The model under review builds one solid part; all positions refer to its coordinate system, in mm. Face numbers are marked on the shaded views. Give positions to 0.01 mm unless a question says otherwise; leave off trailing zeros. Write each loop counter-clockwise with the first axis right and the second up, starting at its lowest first coordinate (ties: lowest second). Pieces come first, ordered by that corner, then holes. Notation, with made-up numbers: (-19.5, -5.75) - (18.5, -5.75) arc R30 cw to (18.5, 22.25) - close; hole circle Ø11 at (-8, -2.5). An arc over 180 degrees is marked (long way). Write item = value, one per line.
```python
from build123d import *

# Parameters (mm, degrees)
SKETCH_1_W          = 140
SKETCH_1_H          = 130
EXTRUDE_1_DEPTH     = 60
CHAMFER_1_SIZE      = 20
SKETCH_2_R          = 50
CUT_EXTRUDE_1_DEPTH = 131
SKETCH_7_R          = 3
CUT_EXTRUDE_2_DEPTH = 61
SKETCH_8_R          = 5.25
CUT_EXTRUDE_3_DEPTH = 35


with BuildPart() as part:
    # 草图1 → 凸台-拉伸1 (new body)
    with BuildSketch(Plane.XY):
        with Locations((70, -65)):
            Rectangle(SKETCH_1_W, SKETCH_1_H)
    extrude(amount=EXTRUDE_1_DEPTH)

    # 倒角1
    chamfer_1_edges = [part.edges().sort_by_distance(p)[0] for p in [
        (140, -65, 60),
        (0, -65, 60),
    ]]
    chamfer(chamfer_1_edges, length=CHAMFER_1_SIZE)

    # 草图2 → 切除-拉伸1 (cut, through all)
    with BuildSketch(Plane(origin=(0, 0, 0), x_dir=(1, 0, 0), z_dir=(0, 1, 0))):
        with Locations((70, 3.2)):
            Circle(SKETCH_2_R)
    extrude(amount=-CUT_EXTRUDE_1_DEPTH, mode=Mode.SUBTRACT)

    # 草图7 → 切除-拉伸2 (cut, through all)
    with BuildSketch(Plane.XY.offset(60)):
        with Locations((7.5, -11)):
            Circle(SKETCH_7_R)
        with Locations((132.5, -11)):
            Circle(SKETCH_7_R)
        with Locations((132.5, -47)):
            Circle(SKETCH_7_R)
        with Locations((132.5, -83)):
            Circle(SKETCH_7_R)
        with Locations((132.5, -119)):
            Circle(SKETCH_7_R)
        with Locations((7.5, -47)):
            Circle(SKETCH_7_R)
        with Locations((7.5, -83)):
            Circle(SKETCH_7_R)
        with Locations((7.5, -119)):
            Circle(SKETCH_7_R)
    extrude(amount=-CUT_EXTRUDE_2_DEPTH, mode=Mode.SUBTRACT)

    # 草图8 → 切除-拉伸3 (cut)
    with BuildSketch(Plane.XY.offset(60)):
        with Locations((7.5, -11)):
            Circle(SKETCH_8_R)
        with Locations((132.5, -11)):
            Circle(SKETCH_8_R)
        with Locations((132.5, -47)):
            Circle(SKETCH_8_R)
        with Locations((132.5, -83)):
            Circle(SKETCH_8_R)
        with Locations((132.5, -119)):
            Circle(SKETCH_8_R)
        with Locations((7.5, -47)):
            Circle(SKETCH_8_R)
        with Locations((7.5, -83)):
            Circle(SKETCH_8_R)
        with Locations((7.5, -119)):
            Circle(SKETCH_8_R)
    extrude(amount=-CUT_EXTRUDE_3_DEPTH, mode=Mode.SUBTRACT)


solid = part.part
```
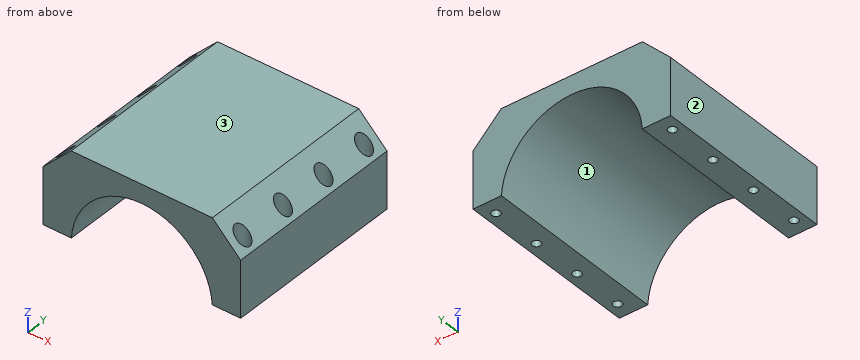
1. Insertion check: P1, Ø1, axis at y = -82, z = 45.5, coming from the +X side; P2, Ø2, axis at x = 44.5, y = -63.5, coming from the -Z side; P3, Ø8.5, axis at x = 7.5, y = -119, coming from the +Z side; P4, Ø4, axis at x = 120, z = 42.5, coming from the +Y side. Each pin has a flat end and moves straight along its axis. Give the tip position at first contact, or say it passes through.
Findings below:
P1 = 127.47
P2 = 39.2
P3 = 25
P4 = 0
2. Take a section at D-D on y = -28. Give the boundary of the cut face in (x, z), and give its area (3 significant figures).
Findings below:
outline = (0, 0) - (20.1, 0) arc R50 cw to (119.9, 0) - (140, 0) - (140, 40) - (120, 60) - (20, 60) - (0, 40) - close
area = 4,390 mm²
3. Take a section at B-B on y = -119. Give the boundary of the cut face in (x, z), and give its area (3 significant figures).
Findings below:
outline = (0, 0) - (4.5, 0) - (4.5, 25) - (2.25, 25) - (2.25, 42.25) - (0, 40) - close; (10.5, 0) - (20.1, 0) arc R50 cw to (119.9, 0) - (129.5, 0) - (129.5, 25) - (127.25, 25) - (127.25, 52.75) - (120, 60) - (20, 60) - (12.75, 52.75) - (12.75, 25) - (10.5, 25) - close; (135.5, 0) - (140, 0) - (140, 40) - (137.75, 42.25) - (137.75, 25) - (135.5, 25) - close
area = 3,620 mm²
4. Draft analysis for pull direction X (two halves, no side actions). For the marked faces 1, 2 and 3, state which applies: +X half, -X half, draft (parallel to the pull), parting line (faces both ways), or undercut.
Findings below:
face_1 = undercut
face_2 = -X half
face_3 = draft
5. For line 1 (Y direction, x = 7.5, z = 16.5); line 2 (Y direction, x = 7.5, z = 31.5); line 3 (X direction, y = -57.5, z = 14.5), list the stretches that pass through material, from the lowest coordinate up. Write a range as from..to.
Findings below:
line_1 = -130..-122, -116..-86, -80..-50, -44..-14, -8..0
line_2 = -130..-124.25, -113.75..-88.25, -77.75..-52.25, -41.75..-16.25, -5.75..0
line_3 = 0..23.24, 116.76..140
6. Take a section at A-A on z = 16. Count the separate pieces of the cut face and the enclosed holes in it, and give its area (3 significant figures).
Findings below:
separate_pieces = 2
enclosed_holes = 8
area = 5,970 mm²
